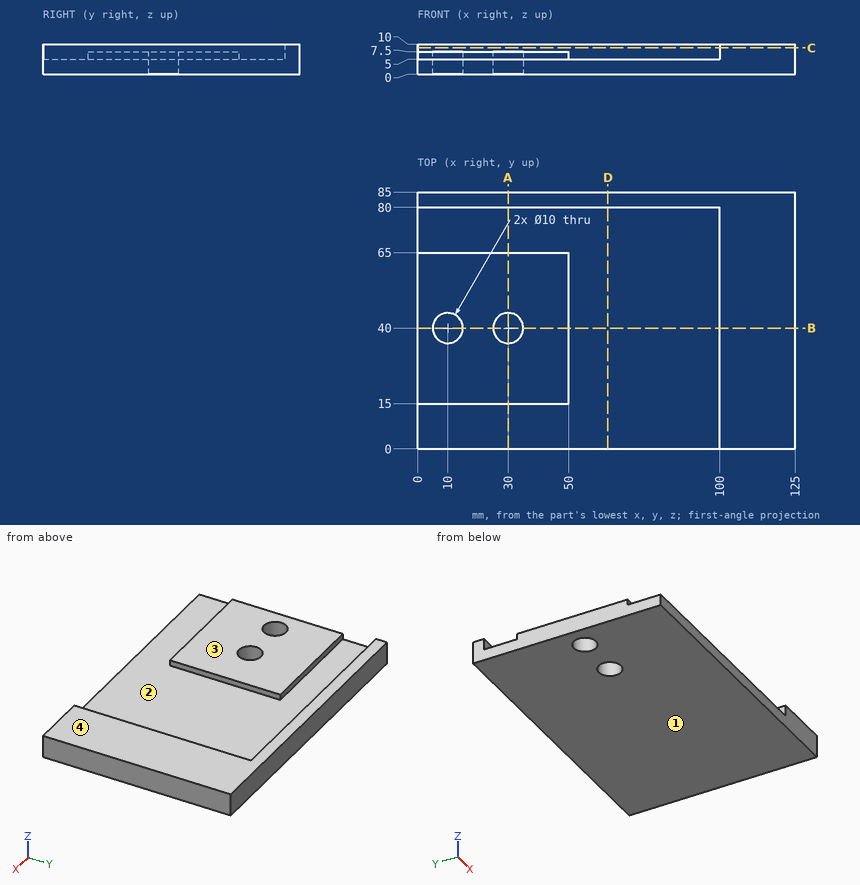
Job drawing, mm, ordinate dimensions from the low corner. One solid piece. A direction names the side the tool comes from. Round coordinates to 2 decimals unless told otherwise and drop trailing zeros. Loops run counter-clockwise (first coordinate to the right, second up) from the corner with the lowest first, then second, coordinate; pieces in that order, holes last.
Item 1: Cut at D-D, the plane x = 63. Give the cut face in (y, z), then the cut area to 3 significant figures.
Item 2: Mould opens along Y. For the marked faces 1 and 2 say: +Y half, -Y half, draft (parallel to the pull), parting line (faces both ways), or undercut.
Item 3: 3-axis set-ups, long thin cutter, end or side, ignore diameter. For the marked faces 3 and 4: which of +Z, -Z, +X, -X, +Y, -Y reach the whole face in a straight line?
Item 4: Drop flat-ended pins along their axis: P1, Ø15, axis at x = 18, y = 49.5, coming from the +Z side; P2, Ø0.8, axis at x = 37, z = 6.5, coming from the -Y side; P3, Ø12, axis at x = 82.5, y = 34, coming from the +Z side. Give the stop position or say it passes through.
Item 5: Cut at A-A, the plane x = 30. Give the cut face in (y, z).
Item 6: Cut at B-B, the plane y = 40. Give the cut face in (x, z), then the cut area to 3 significant figures.
Item 7: Drill centre lines: line 1 (Y direction, x = 30, z = 6); line 2 (Y direction, x = 9.5, z = 4.25); line 3 (Y direction, x = 34, z = 6). Where is each one in solid material? Low to high.
Item 8: Cut at C-C, the plane z = 8.75. Give the cut face in (x, y).
A:
1. outline: (0, 0) - (85, 0) - (85, 10) - (80, 10) - (80, 5) - (0, 5) - close
1. area: 450 mm2
2. face 1: draft
2. face 2: undercut
3. face 3: +Z, -X, -Y
3. face 4: +Z, +X, -X, +Y, -Y
4. P1: stops at z = 7.5
4. P2: stops at y = 15
4. P3: stops at z = 5
5. outline: (0, 0) - (35, 0) - (35, 7.5) - (15, 7.5) - (15, 5) - (0, 5) - close; (45, 0) - (85, 0) - (85, 10) - (80, 10) - (80, 5) - (65, 5) - (65, 7.5) - (45, 7.5) - close
6. outline: (0, 0) - (5, 0) - (5, 7.5) - (0, 7.5) - close; (15, 0) - (25, 0) - (25, 7.5) - (15, 7.5) - close; (35, 0) - (125, 0) - (125, 10) - (100, 10) - (100, 5) - (50, 5) - (50, 7.5) - (35, 7.5) - close
6. area: 725 mm2
7. line 1: y = 15 to 35, 45 to 65, 80 to 85
7. line 2: y = 0 to 35.03, 44.97 to 85
7. line 3: y = 15 to 37, 43 to 65, 80 to 85
8. outline: (0, 80) - (100, 80) - (100, 0) - (125, 0) - (125, 85) - (0, 85) - close
